CAD build for the part. Positions are in the model's coordinates, mm. Round coordinates to 2 decimals unless told otherwise and drop trailing zeros. Order: outer loops, then holes, each group sorted by start corner. A loop starts at its lowest first (then second) coordinate and runs counter-clockwise, first axis right, second up. Notation, with made-up numbers: M 4,49.5 L 31,49.5 A23 ccw 31,87.5 Z; hole C 81.25,9 d9. An arc over 180 degrees is marked long. Answer as a JSON object with one key per item and string values.
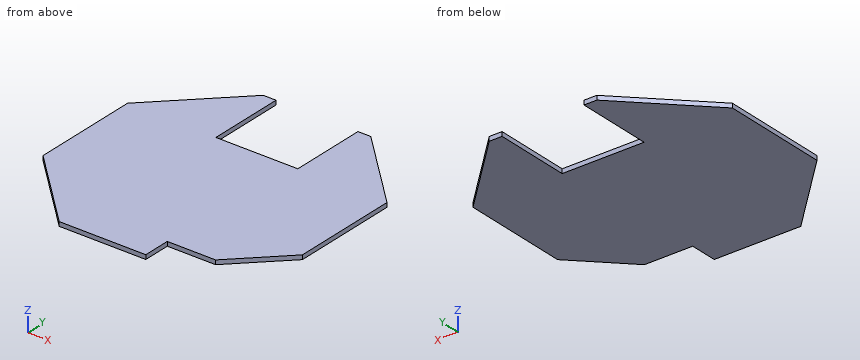
Autodesk Inventor part; units mm, degrees
ref_plane "YZ Plane" through (0, 0, 0) normal (1, 0, 0) x (0, 1, 0)
ref_plane "XZ Plane" through (0, 0, 0) normal (0, 1, 0) x (-1, 0, 0)
ref_plane "XY Plane" through (0, 0, 0) normal (0, 0, 1) x (1, 0, 0)
sketch "Sketch1" plane through (0, 0, 0) normal (0, 0, 1) x (1, 0, 0)
  line L0 (0, 0) -> (0, 24.8008)
  line L1 (0, 0) -> (23.5103, 0)
  line L2 (-19.7, 47.5) -> (19.7, 47.5)
  line L3 (47.5, 19.7) -> (47.5, -19.7)
  line L4 (19.7, -47.5) -> (-19.7, -47.5)
  line L5 (-47.5, -19.7) -> (-47.5, 19.7)
  line L6 (19.7, 47.5) -> (47.5, 19.7)
  line L7 (47.5, -19.7) -> (19.7, -47.5)
  line L8 (-19.7, -47.5) -> (-47.5, -19.7)
  line L9 (-47.5, 19.7) -> (-19.7, 47.5)
  point P0 (-47.5, 47.5)
  point P1 (47.5, -47.5)
  point P2 (47.5, 47.5)
  point P3 (-47.5, -47.5)
  dimension "d9" = 27.8
  dimension "d10" = 27.8
  dimension "d11" = 27.8
  dimension "d12" = 27.8
  dimension "d13" = 27.8
  dimension "d14" = 27.8
  dimension "d15" = 27.8
  dimension "d16" = 27.8
  dimension "d17" = 95
  dimension "d18" = 95
extrude "Extrusion1" add sketch "Sketch1" along normal mid plane 1.5748
sketch "Sketch2" plane through (0, 0, 0.7874) normal (0, 0, 1) x (1, 0, 0)
  line L0 (0, 0) -> (0, 42.1348)
  line L1 (-15, 47.5) -> (15, 47.5)
  line L2 (15, 47.5) -> (15, 19.5)
  line L3 (15, 19.5) -> (-15, 19.5)
  line L4 (-15, 19.5) -> (-15, 47.5)
  line L5 (-19.7, 47.5) -> (19.7, 47.5)
  dimension "d4" = 30
  dimension "d25" = 28
extrude "Extrusion2" cut sketch "Sketch2" against normal through all
sketch "Sketch3" plane through (0, 0, 0.7874) normal (0, 0, 1) x (1, 0, 0)
  line L0 (19.7, -47.5) -> (-19.7, -47.5)
  line L1 (12, -47.5) -> (32, -47.5)
  line L2 (32, -47.5) -> (32, -37.5)
  line L3 (32, -37.5) -> (12, -37.5)
  line L4 (12, -37.5) -> (12, -47.5)
  point P0 (0, 0)
  dimension "d19" = 10
  dimension "d21" = 12
  dimension "d24" = 32
extrude "Extrusion3" cut sketch "Sketch3" against normal through all
properties part number "Tant_Exp4_top" material "Lead"
Item 1: Saw through at D-D on x = 33.5. List the corners of the cut face in (y, z), and give its area (3 significant figures).
Worked answers:
{"outline": "M -33.7,-0.79 L 33.7,-0.79 L 33.7,0.79 L -33.7,0.79 Z", "area": "106 mm2"}
Item 2: Saw through at A-A on y = 39. List the corners of the cut face in (x, z).
Worked answers:
{"outline": "M -28.2,-0.79 L -15,-0.79 L -15,0.79 L -28.2,0.79 Z; M 15,-0.79 L 28.2,-0.79 L 28.2,0.79 L 15,0.79 Z"}
Item 3: Saw through at B-B on z = -0.05. List the corners of the cut face in (x, y).
Worked answers:
{"outline": "M -47.5,-19.7 L -19.7,-47.5 L 12,-47.5 L 12,-37.5 L 29.7,-37.5 L 47.5,-19.7 L 47.5,19.7 L 19.7,47.5 L 15,47.5 L 15,19.5 L -15,19.5 L -15,47.5 L -19.7,47.5 L -47.5,19.7 Z"}
Item 4: Drop a flat-ended pin along its axis: pin 1 Ø0.8 at (x, z) = (6, 0) entering from +Y. Give the stop position or say it passes through.
Worked answers:
{"pin 1": "stops at y = 19.5"}
Item 5: Wall check: line 1 along Y through (x, z) = (5, -0.7); line 2 along X through (y, z) = (34, 0.05); line 3 along X through (y, z) = (20, 0.2). Give the ranges that are in metal, low to high. Write a range as [from, to].
Worked answers:
{"line 1": "y = [-47.5, 19.5]", "line 2": "x = [-33.2, -15], [15, 33.2]", "line 3": "x = [-47.2, -15], [15, 47.2]"}
Item 6: Saw through at C-C on y = 29. List the corners of the cut face in (x, z), and give its area (3 significant figures).
Worked answers:
{"outline": "M -38.2,-0.79 L -15,-0.79 L -15,0.79 L -38.2,0.79 Z; M 15,-0.79 L 38.2,-0.79 L 38.2,0.79 L 15,0.79 Z", "area": "73.1 mm2"}
